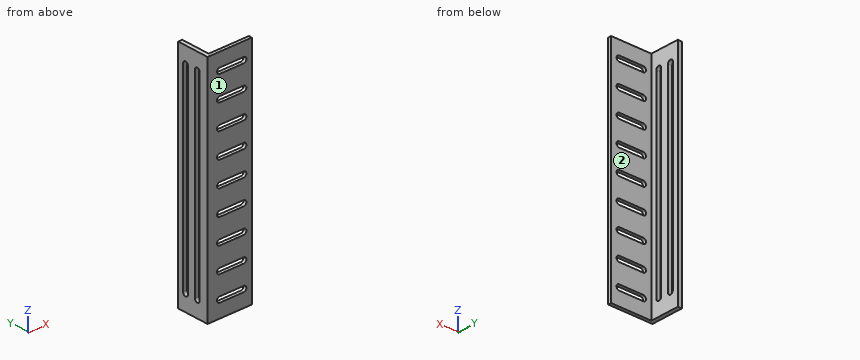
Autodesk Inventor part; units mm, degrees
ref_plane "YZ Plane" through (0, 0, 0) normal (1, 0, 0) x (0, 1, 0)
ref_plane "XZ Plane" through (0, 0, 0) normal (0, 1, 0) x (-1, 0, 0)
ref_plane "XY Plane" through (0, 0, 0) normal (0, 0, 1) x (1, 0, 0)
sketch "Sketch1" plane through (0, 0, 0) normal (0, 1, 0) x (-1, 0, 0)
  line L0 (0, 0) -> (-27.5, 0)
  line L1 (-27.5, 0) -> (-27.5, -140)
  line L2 (-27.5, -140) -> (0, -140)
  line L3 (0, -140) -> (0, 0)
  line L4 (0, 0) -> (-2.5, 0)
  line L5 (-2.5, 0) -> (-2.5, -140)
  line L6 (-2.5, -140) -> (0, -140)
  line L7 (0, -140) -> (0, 0)
  arc A0 (-7.5, -11.65) -> (-7.5, -8.35) centre (-7.5, -10) ccw
  arc A1 (-22.5, -8.35) -> (-22.5, -11.65) centre (-22.5, -10) ccw
  line L8 (-7.5, -11.65) -> (-22.5, -11.65)
  line L9 (-22.5, -8.35) -> (-7.5, -8.35)
  arc A2 (-7.5, -26.65) -> (-7.5, -23.35) centre (-7.5, -25) ccw
  line L10 (-22.5, -23.35) -> (-7.5, -23.35)
  line L11 (-7.5, -26.65) -> (-22.5, -26.65)
  arc A3 (-22.5, -23.35) -> (-22.5, -26.65) centre (-22.5, -25) ccw
  arc A4 (-7.5, -41.65) -> (-7.5, -38.35) centre (-7.5, -40) ccw
  line L12 (-22.5, -38.35) -> (-7.5, -38.35)
  line L13 (-7.5, -41.65) -> (-22.5, -41.65)
  arc A5 (-22.5, -38.35) -> (-22.5, -41.65) centre (-22.5, -40) ccw
  arc A6 (-7.5, -56.65) -> (-7.5, -53.35) centre (-7.5, -55) ccw
  line L14 (-22.5, -53.35) -> (-7.5, -53.35)
  line L15 (-7.5, -56.65) -> (-22.5, -56.65)
  arc A7 (-22.5, -53.35) -> (-22.5, -56.65) centre (-22.5, -55) ccw
  arc A8 (-7.5, -71.65) -> (-7.5, -68.35) centre (-7.5, -70) ccw
  line L16 (-22.5, -68.35) -> (-7.5, -68.35)
  line L17 (-7.5, -71.65) -> (-22.5, -71.65)
  arc A9 (-22.5, -68.35) -> (-22.5, -71.65) centre (-22.5, -70) ccw
  arc A10 (-7.5, -86.65) -> (-7.5, -83.35) centre (-7.5, -85) ccw
  line L18 (-22.5, -83.35) -> (-7.5, -83.35)
  line L19 (-7.5, -86.65) -> (-22.5, -86.65)
  arc A11 (-22.5, -83.35) -> (-22.5, -86.65) centre (-22.5, -85) ccw
  arc A12 (-7.5, -101.65) -> (-7.5, -98.35) centre (-7.5, -100) ccw
  line L20 (-22.5, -98.35) -> (-7.5, -98.35)
  line L21 (-7.5, -101.65) -> (-22.5, -101.65)
  arc A13 (-22.5, -98.35) -> (-22.5, -101.65) centre (-22.5, -100) ccw
  arc A14 (-7.5, -116.65) -> (-7.5, -113.35) centre (-7.5, -115) ccw
  line L22 (-22.5, -113.35) -> (-7.5, -113.35)
  line L23 (-7.5, -116.65) -> (-22.5, -116.65)
  arc A15 (-22.5, -113.35) -> (-22.5, -116.65) centre (-22.5, -115) ccw
  arc A16 (-7.5, -131.65) -> (-7.5, -128.35) centre (-7.5, -130) ccw
  line L24 (-22.5, -128.35) -> (-7.5, -128.35)
  line L25 (-7.5, -131.65) -> (-22.5, -131.65)
  arc A17 (-22.5, -128.35) -> (-22.5, -131.65) centre (-22.5, -130) ccw
  dimension "d0" = 27.5
  dimension "d1" = 140
  dimension "d2" = 2.5
  dimension "d21" = 3.3
  dimension "d22" = 10
  dimension "d23" = 5
  dimension "d24" = 3.3
  dimension "d25" = 5
  dimension "d28" = 15
extrude "Extrusion1" add sketch "Sketch1" along normal blind 2 contours L5 L2 L1 L0
extrude "Extrusion2" add sketch "Sketch1" along normal blind 20 contours L3 L2 L5 L0
sketch "Sketch2" plane through (2.5, 2, -140) normal (1, 0, 0) x (0, 0, -1)
  circle A0 centre (-130, 5) radius 1.65
  line L0 (0, 0) -> (-140, 0)
  circle A1 centre (-130, 13) radius 1.65
  line L1 (-140, 18) -> (0, 18)
  line L2 (-140, 0) -> (-140, 18)
  line L3 (0, 0) -> (0, 18)
  line L4 (-130, 13) -> (-10, 13) construction
  line L5 (-130, 11.35) -> (-10, 11.35)
  line L6 (-10, 14.65) -> (-130, 14.65)
  arc A2 (-130, 14.65) -> (-130, 11.35) centre (-130, 13) ccw
  arc A3 (-10, 11.35) -> (-10, 14.65) centre (-10, 13) ccw
  line L7 (-130, 5) -> (-10, 5) construction
  line L8 (-130, 3.35) -> (-10, 3.35)
  line L9 (-10, 6.65) -> (-130, 6.65)
  arc A4 (-130, 6.65) -> (-130, 3.35) centre (-130, 5) ccw
  arc A5 (-10, 3.35) -> (-10, 6.65) centre (-10, 5) ccw
  point P0 (-140, -2)
  point P1 (-70, 13)
  point P2 (-70, 5)
  point P3 (-130, 6.65)
  point P4 (-130, 3.35)
  point P5 (-130, 14.65)
  point P6 (-130, 11.35)
  dimension "d7" = 3.3
  dimension "d8" = 5
  dimension "d9" = 3.3
  dimension "d10" = 5
  dimension "d11" = 10
  dimension "d12" = 10
  dimension "d15" = 3.3
  dimension "d16" = 3.3
  dimension "d19" = 120
  dimension "d20" = 120
extrude "Extrusion3" cut sketch "Sketch2" against normal blind 2.5 contours A0 | A0 L9 A5 L8 | A1 | A1 L6 A3 L5
properties part number "Alas Conveyor_3DPrint"
Model file for the job. Use its own axes, mm. Face numbers are marked on the shaded views. A direction names the side the tool comes from. Coordinates: 2 decimals unless noted, no trailing zeros. Write each loop counter-clockwise with the first axis right and the second up, starting at its lowest first coordinate (ties: lowest second). Pieces come first, ordered by that corner, then holes. Notation, with made-up numbers: (41.25, 79.25) - (91.25, 79.25) arc R24 cw to (91.25, 116.25) - close; hole circle Ø2 at (-37, 1.5). An arc over 180 degrees is marked (long way). One line per item, written item: value. Start each with the question number.
1. Flat gauge pins, fed straight in: pin 1 (8 mm diameter, centred on x = 9, y = 7, fed in from +Z); pin 2 (4 mm diameter, centred on x = 14.5, z = -62, fed in from +Y); pin 3 (1.5 mm diameter, centred on y = 16, z = -73, fed in from +X). Where does each tip first touch, or does it go through?
2. Slice it at B-B (y = 7). Write the cut outline in (x, z), plus the area to 4 significant figures.
3. Slice it at A-A (z = -85). Write the cut outline in (x, y), plus the area to 3 significant figures.
4. Tool access for the marked faces 1 and 2: list every direction of +Z, -Z, +X, -X, +Y, -Y with a clear straight run to the whole face (end or side of a thin tool).
5. Probe line 1 (Y direction, x = 1.5, z = -45.5); line 2 (Y direction, x = 20.75, z = -48); line 3 (X direction, y = 2.5, z = -111.5). List the from-to ranges inside material, lowest first. Write a range as from..to.
6. Slice it at D-D (x = 10.75). Count the separate pieces of the cut face and the enclosed holes in it, plus the area to 3 significant figures.
7. Slice it at C-C (z = -49.5). Write the cut outline in (x, y), plus the area to 3 significant figures.
Answers below:
1. pin 1: passes through
1. pin 2: stops at y = 2
1. pin 3: stops at x = 2.5
2. outline: (0, -140) - (2.5, -140) - (2.5, -131.65) - (0, -131.65) - close; (0, -8.35) - (2.5, -8.35) - (2.5, 0) - (0, 0) - close
2. area: 41.75 mm^2
3. outline: (0, 0) - (5.85, 0) - (5.85, 2) - (2.5, 2) - (2.5, 5.35) - (0, 5.35) - close; (0, 8.65) - (2.5, 8.65) - (2.5, 13.35) - (0, 13.35) - close; (0, 16.65) - (2.5, 16.65) - (2.5, 20) - (0, 20) - close; (24.15, 0) - (27.5, 0) - (27.5, 2) - (24.15, 2) - close
3. area: 46.9 mm^2
4. face 1: +Z, -Z, +X, -X, -Y
4. face 2: +Z, -Z, +X, +Y
5. line 1: y = 0..5.35, 8.65..13.35, 16.65..20
5. line 2: y = 0..2
5. line 3: x = 0..2.5
6. separate pieces: 10
6. enclosed holes: 0
6. area: 221 mm^2
7. outline: (0, 0) - (27.5, 0) - (27.5, 2) - (2.5, 2) - (2.5, 5.35) - (0, 5.35) - close; (0, 8.65) - (2.5, 8.65) - (2.5, 13.35) - (0, 13.35) - close; (0, 16.65) - (2.5, 16.65) - (2.5, 20) - (0, 20) - close
7. area: 83.5 mm^2
